from build123d import *

# Parameters (mm, degrees)
SKETCH_1_R          = 1.35
SKETCH_1_R_2        = 1.6
EXTRUDE_1_DEPTH     = 1.5
FILLET_1_R          = 3
CUT_EXTRUDE_1_DEPTH = 6.5
FILLET_2_R          = 1.5


with BuildPart() as part:
    # 草图1 → 凸台-拉伸1 (new, symmetric)
    with BuildSketch(Plane.XY):
        Polygon((-110, 18.502065587), (-110, -18.502065587), (-23.765491901, -30), (23.765491901, -30), (110, -18.502065587), (110, 18.502065587), (23.765491901, 30), (-23.765491901, 30), align=None)
        with Locations((-31, 25)):
            Circle(SKETCH_1_R, mode=Mode.SUBTRACT)
        with Locations((31, 25)):
            Circle(SKETCH_1_R, mode=Mode.SUBTRACT)
        with Locations((-31, -25)):
            Circle(SKETCH_1_R, mode=Mode.SUBTRACT)
        with Locations((31, -25)):
            Circle(SKETCH_1_R, mode=Mode.SUBTRACT)
        with Locations((-106, 15)):
            Circle(SKETCH_1_R_2, mode=Mode.SUBTRACT)
        with Locations((-106, -15)):
            Circle(SKETCH_1_R_2, mode=Mode.SUBTRACT)
        with Locations(Location((106, -15, 0), (0, 0, 180))):
            Circle(SKETCH_1_R_2, mode=Mode.SUBTRACT)
        with Locations(Location((106, 15, 0), (0, 0, 180))):
            Circle(SKETCH_1_R_2, mode=Mode.SUBTRACT)
    extrude(amount=EXTRUDE_1_DEPTH, both=True)

    # 圆角1
    fillet_1_edges = [part.edges().sort_by_distance(p)[0] for p in [
        (23.765491901, -30, 0),
        (-23.765491901, -30, 0),
        (-110, -18.502065587, 0),
        (-110, 18.502065587, 0),
        (-23.765491901, 30, 0),
        (23.765491901, 30, 0),
        (110, 18.502065587, 0),
        (110, -18.502065587, 0),
    ]]
    fillet(fillet_1_edges, radius=FILLET_1_R)

    # 草图2 → 切除-拉伸1 (cut, symmetric)
    with BuildSketch(Plane.XY.offset(1.5)):
        Polygon((-99.293086989, 11.858856148), (-78.133261722, 1.66499219), (-40.778661074, 19.660779603), align=None)
        Polygon((-74.677168531, 0), (-35.999998999, -18.632942356), (-35.999998999, 18.632942356), align=None)
        Polygon((-99.293086989, -11.858856148), (-40.778661074, -19.660779603), (-78.133261722, -1.66499219), align=None)
        Polygon((-102, -9.832942223), (-81.589354914, 0), (-102, 9.832942223), align=None)
        Polygon((-30.999998999, 20.160653741), (-30.999998999, -20.160653741), (-2.591806009, 0), align=None)
        Polygon((-28.40819299, 22), (0, 1.839346259), (28.40819299, 22), align=None)
        Polygon((30.999998999, 20.160653741), (2.591806009, 0), (30.999998999, -20.160653741), align=None)
        Polygon((0, -1.839346259), (-28.40819299, -22), (28.40819299, -22), align=None)
        Polygon((35.999998999, -18.632942356), (74.677168531, 0), (35.999998999, 18.632942356), align=None)
        Polygon((78.133261722, 1.66499219), (99.293086989, 11.858856148), (40.778661074, 19.660779603), align=None)
        Polygon((102, 9.832942223), (81.589354914, 0), (102, -9.832942223), align=None)
        Polygon((99.293086989, -11.858856148), (78.133261722, -1.66499219), (40.778661074, -19.660779603), align=None)
    extrude(amount=CUT_EXTRUDE_1_DEPTH, both=True, mode=Mode.SUBTRACT)

    # 圆角2
    fillet_2_edges = [part.edges().sort_by_distance(p)[0] for p in [
        (2.591806009, 0, 0),
        (30.999998999, 20.160653741, 0),
        (30.999998999, -20.160653741, 0),
        (0, 1.839346259, 0),
        (-28.40819299, 22, 0),
        (28.40819299, 22, 0),
        (-28.40819299, -22, 0),
        (0, -1.839346259, 0),
        (28.40819299, -22, 0),
        (35.999998999, -18.632942356, 0),
        (35.999998999, 18.632942356, 0),
        (74.677168531, 0, 0),
        (-78.133261722, -1.66499219, 0),
        (-40.778661074, -19.660779603, 0),
        (-99.293086989, -11.858856148, 0),
        (-74.677168531, 0, 0),
        (-35.999998999, 18.632942356, 0),
        (-35.999998999, -18.632942356, 0),
        (-102, -9.832942223, 0),
        (-102, 9.832942223, 0),
        (-81.589354914, 0, 0),
        (-30.999998999, -20.160653741, 0),
        (-30.999998999, 20.160653741, 0),
        (-2.591806009, 0, 0),
        (40.778661074, -19.660779603, 0),
        (78.133261722, -1.66499219, 0),
        (99.293086989, -11.858856148, 0),
        (40.778661074, 19.660779603, 0),
        (99.293086989, 11.858856148, 0),
        (78.133261722, 1.66499219, 0),
        (102, 9.832942223, 0),
        (102, -9.832942223, 0),
        (81.589354914, 0, 0),
        (-99.293086989, 11.858856148, 0),
        (-40.778661074, 19.660779603, 0),
        (-78.133261722, 1.66499219, 0),
    ]]
    fillet(fillet_2_edges, radius=FILLET_2_R)


solid = part.part
Model file for the job. Use its own axes, mm. A direction names the side the tool comes from. Give positions to 0.01 mm unless a question says otherwise; leave off trailing zeros. Order: outer loops, then holes, each group sorted by start corner. A loop starts at its lowest first (then second) coordinate and runs counter-clockwise, first axis right, second up. Notation, with made-up numbers: M 5,42.25 L 43,42.25 A17 cw 43,68.25 Z; hole C 25.5,12 d10. An arc over 180 degrees is marked long. Write item = value, one per line.
Q1. Tool access for faces 4 (the flat face through (16.64, 9.97, -0.02)), 5 (the flat face through (66.264, 24.334, 0.021)): list every direction of +Z, -Z, +X, -X, +Y, -Y with a clear straight run to the whole face (end or side of a thin tool).
Derived:
face_4 = +Z, -Z
face_5 = +Z, -Z, +X, +Y
Q2. Flat gauge pins, fed straight in: pin 1 (8 mm diameter, centred on x = -24, y = -10.5, fed in from +Z); pin 2 (1 mm diameter, centred on x = -50.5, z = -0.5, fed in from +Y). Where does each tip first touch, or does it go through?
Derived:
pin_1 = 1.5
pin_2 = 26.5
Q3. Cut at A-A, the plane x = 68.5. List the corners of the cut face in (y, z).
Derived:
outline = M -24.04,-1.5 L -15.96,-1.5 L -15.96,1.5 L -24.04,1.5 Z; M -6.31,-1.5 L -2.98,-1.5 L -2.98,1.5 L -6.31,1.5 Z; M 2.98,-1.5 L 6.31,-1.5 L 6.31,1.5 L 2.98,1.5 Z; M 15.96,-1.5 L 24.04,-1.5 L 24.04,1.5 L 15.96,1.5 Z
Q4. Two-plate mould, pull along Y, no slides. Class faces 1 (the flat face through (-86.893, 5.885, -0.021)), 2 (the flat face through (-65.1, 24.49, 0.02)), 3 (the flat face through (-66.264, -24.334, 0.021)): pulls with the +Y half, pulls with the -Y half, needs draft (parallel to the pull), parting line crosses it, or undercut.
Derived:
face_1 = undercut
face_2 = pulls with the +Y half
face_3 = pulls with the -Y half
Q5. Cut at B-B, the plane x = -43.5. List the corners of the cut face in (y, z), then the cut area to 3 significant figures.
Derived:
outline = M -27.37,-1.5 L -15.02,-1.5 L -15.02,1.5 L -27.37,1.5 Z; M 15.02,-1.5 L 27.37,-1.5 L 27.37,1.5 L 15.02,1.5 Z
area = 74.1 mm2
Q6. Drill centre lines: line 1 (X direction, y = 18.5, z = -0.05); line 2 (Y direction, x = -106, z = -0.75); line 3 (Y direction, x = -62, z = -0.15). Where is each one in solid material? Low to high. Write a range as [from, to].
Derived:
line_1 = [-108.45, -30.34], [-28.66, -23.48], [23.48, 28.66], [30.34, 108.45]
line_2 = [-19.04, -16.6], [-13.4, 13.4], [16.6, 19.04]
line_3 = [-24.9, -16.83], [-9.44, -6.11], [6.11, 9.44], [16.83, 24.9]
Q7. Cut at C-C, the plane z = 0.3. Count the separate pieces of the cut face and the enclosed holes in it, then the cut area to 3 significant figures.
Derived:
separate_pieces = 1
enclosed_holes = 20
area = 5,610 mm2
Q8. Cut at D-D, the plane x = -19.5. List the corners of the cut face in (y, z), then the cut area to 3 significant figures.
Derived:
outline = M -30,-1.5 L -22,-1.5 L -22,1.5 L -30,1.5 Z; M -15.68,-1.5 L -12,-1.5 L -12,1.5 L -15.68,1.5 Z; M 12,-1.5 L 15.68,-1.5 L 15.68,1.5 L 12,1.5 Z; M 22,-1.5 L 30,-1.5 L 30,1.5 L 22,1.5 Z
area = 70.1 mm2
